The listing builds one solid part. Answer for the finished solid, in the listing's coordinates (mm). A direction names the side the tool comes from. Coordinates: 2 decimals unless noted, no trailing zeros. Loops run counter-clockwise (first coordinate to the right, second up) from the corner with the lowest first, then second, coordinate; pieces in that order, holes last. Notation, with made-up numbers: M 57.25,16.25 L 80.25,16.25 A8 ccw 80.25,20.25 Z; hole C 68,-30.75 d7. An arc over 180 degrees is marked long. Return JSON: item names as keys, results as strings. Group by question number.
1. Which of the six approach directions +Z, -Z, +X, -X, +Y, -Y give full straight-line access (tool end or side, diameter ignored) to faces 5 (the face through (0, -19, -21.788)), 6 (the face through (0, -1, 0))?
2. Given P1, Ø3.5, axis at x = -20, z = -18.46, coming from the -Y side; P2, Ø3, axis at x = 20, y = 11, coming from the -Z side; P3, Ø10.5, axis at x = -6, z = -8, coming from the +Y side, each flat-ended and moving along its own axis, determine where each tip first touches the part or whether it passes through.
3. Section B-B (y = 9) is taken. Write down the section's boundary in (x, z), then the cut area to 3 significant figures.
4. Section A-A (x = -13.15) is taken. Write down the section's boundary in (y, z), then the cut area to 3 significant figures.
5. Straight lines are drawn through the part: L1, parallel to Y at x = -3.5, z = -8; L2, parallel to Z at x = -6.5, y = -10; L3, parallel to Y at x = -13.15, z = 1.5. For each, find the intervals that lie inside material, in ascending order. Write a range as from..to.
6. Section C-C (z = -3.25) is taken. Write down the section's boundary in (x, y), then the cut area to 3 significant figures.
7. The mould has two halves that part along Y. Classify faces 1 (the face through (-21, 3, 1)), 2 (the face through (0, -1, 2)), 3 (the face through (-0.35, -19.2, 1.14)), 4 (the face through (0.35, -17.799, -0.285)): pulls with the +Y half, pulls with the -Y half, needs draft (parallel to the pull), parting line crosses it, or undercut.
8. Section D-D (x = -4.5) is taken. Write down the section's boundary in (y, z).
```python
from build123d import *

# Parameters (mm, degrees)
SKETCH1_W           = 50
SKETCH1_H           = 30
SKETCH1_R           = 8.1
BOSS_EXTRUDE1_DEPTH = 2
SKETCH3_W           = 50
SKETCH3_H           = 2
SKETCH5_R           = 2
CUT_EXTRUDE1_DEPTH  = 47.853803709


with BuildPart() as part:
    # Sketch1 → Boss-Extrude1 (new body)
    with BuildSketch(Plane.XY):
        Rectangle(SKETCH1_W, SKETCH1_H)
        with Locations((13.15, 5)):
            Circle(SKETCH1_R, mode=Mode.SUBTRACT)
        with Locations(Location((-13.15, 5, 0), (0, 0, 180))):
            Circle(SKETCH1_R, mode=Mode.SUBTRACT)
    extrude(amount=BOSS_EXTRUDE1_DEPTH)

    # Sweep1: sweep along a path in Sketch2
    with BuildLine(Plane(origin=(25, 0, 0), x_dir=(0, 0, -1), z_dir=(1, 0, 0))) as sweep1_path:
        Line((-1, -15), (-1, -17.099519782))
        ThreePointArc((-1, -17.099519782), (-0.414213562, -18.513733344), (1, -19.099519782))
        Line((1, -19.099519782), (21.787627504, -19.099519782))
    # Sketch3 → Sweep1 (sweep)
    with BuildSketch(Plane.XZ.offset(15)):
        with Locations((0, 1)):
            Rectangle(SKETCH3_W, SKETCH3_H)
    sweep(path=sweep1_path.line)

    # Sketch5 → Cut-Extrude1 (cut, through all)
    with BuildSketch(Plane(origin=(0, -18.099519782, 0), x_dir=(1, 0, 0), z_dir=(0, 1, 0))):
        with Locations(Location((-20, 18.460437776, 0), (0, 0, 270))):
            Circle(SKETCH5_R)
        with Locations(Location((20, 18.460437776, 0), (0, 0, 90))):
            Circle(SKETCH5_R)
    extrude(amount=-CUT_EXTRUDE1_DEPTH, mode=Mode.SUBTRACT)


solid = part.part
```
Worked out:
{
 "1": {"face 5": "-Z, +X, -X, +Y, -Y", "face 6": "-Z, +X, -X, +Y"},
 "2": {"P1": "through", "P2": "z = 0", "P3": "y = -18.1"},
 "3": {"outline": "M -25,0 L -20.19,0 L -20.19,2 L -25,2 Z; M -6.11,0 L 6.11,0 L 6.11,2 L -6.11,2 Z; M 20.19,0 L 25,0 L 25,2 L 20.19,2 Z", "area": "43.7 mm^2"},
 "4": {"outline": "M -20.1,-21.79 L -18.1,-21.79 L -18.1,-1 A1 cw -17.1,0 L -3.1,0 L -3.1,2 L -17.1,2 A3 ccw -20.1,-1 Z; M 13.1,0 L 15,0 L 15,2 L 13.1,2 Z", "area": "79.7 mm^2"},
 "5": {"L1": "-20.1..-18.1", "L2": "0..2", "L3": "-18.76..-3.1, 13.1..15"},
 "6": {"outline": "M -25,-20.1 L 25,-20.1 L 25,-18.1 L -25,-18.1 Z", "area": "100 mm^2"},
 "7": {"face 1": "undercut", "face 2": "needs draft", "face 3": "pulls with the -Y half", "face 4": "pulls with the +Y half"},
 "8": {"outline": "M -20.1,-21.79 L -18.1,-21.79 L -18.1,-1 A1 cw -17.1,0 L 15,0 L 15,2 L -17.1,2 A3 ccw -20.1,-1 Z"}
}
